Geometry: see drawing. Coordinates: mm, zero at the bounding-box minimum. A direction names the side the tool comes from. Give positions to 0.01 mm unless a question says otherwise; leave off trailing zeros. Order: outer loops, then holes, each group sorted by start corner. A loop starts at its lowest first (then second) coordinate and runs counter-clockwise, first axis right, second up. Notation, with made-up numbers: (-0.5, 15) -> (16.5, 15) arc R20 ccw to (16.5, 40) -> close; hole circle Ø2 at (22.5, -25.75). An arc over 180 degrees is marked (long way). Use one line per item in the form item = value. Start each with the question number.
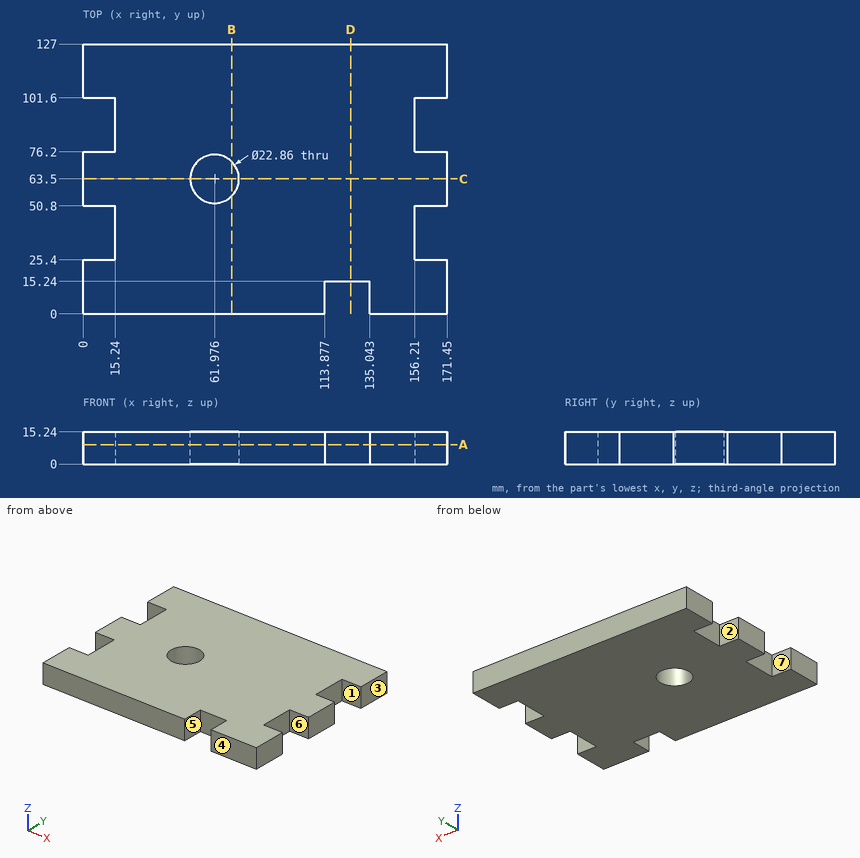
1) Cut plane A-A, the plane z = 9.25. Return the cut outline in (x, y).
2) Draft query along Y for the marked faces 1, 2, 3 and 4. Return one class per face: +Y half, -Y half, draft (parallel to the pull), parting line (faces both ways), or undercut.
3) Pin query (flat end, axial travel): pin 1 (1.5 mm diameter, centred on x = 37.5, z = 6.5, fed in from -Y); pin 2 (4.5 mm diameter, centred on y = 32.5, z = 4.5, fed in from -X); pin 3 (7.5 mm diameter, centred on y = 89, z = 11, fed in from +X). Return the tip coordinate at first contact, or that it passes through.
4) Cut plane D-D, the plane x = 126. Return the cut outline in (y, z).
5) Material intervals for probe 1 along Y at (x, z) = (8.5, 1.5); probe 2 along X at (y, z) = (81.5, 13.75); probe 3 along Y at (x, z) = (116, 7.25), sorted ascending.
6) Reachability of the marked faces 5, 6 and 7 from +Z, -Z, +X, -X, +Y, -Y: full face, straight path, thin tool, end or side. Return the list, or none.
7) Cut plane B-B, the plane x = 70. Return the cut outline in (y, z), plus the area to 3 significant figures.
8) Cut plane C-C, the plane y = 63.5. Return the cut outline in (x, z).
Output values:
q1.outline = (0, 0) -> (113.88, 0) -> (113.88, 15.24) -> (135.04, 15.24) -> (135.04, 0) -> (171.45, 0) -> (171.45, 25.4) -> (156.21, 25.4) -> (156.21, 50.8) -> (171.45, 50.8) -> (171.45, 76.2) -> (156.21, 76.2) -> (156.21, 101.6) -> (171.45, 101.6) -> (171.45, 127) -> (0, 127) -> (0, 101.6) -> (15.24, 101.6) -> (15.24, 76.2) -> (0, 76.2) -> (0, 50.8) -> (15.24, 50.8) -> (15.24, 25.4) -> (0, 25.4) -> close; hole circle Ø22.86 at (61.98, 63.5)
q2.face_1 = undercut
q2.face_2 = undercut
q2.face_3 = draft
q2.face_4 = -Y half
q3.pin_1 = 0
q3.pin_2 = 15.24
q3.pin_3 = 156.21
q4.outline = (15.24, 0) -> (127, 0) -> (127, 15.24) -> (15.24, 15.24) -> close
q5.probe_1 = 0 to 25.4, 50.8 to 76.2, 101.6 to 127
q5.probe_2 = 15.24 to 156.21
q5.probe_3 = 15.24 to 127
q6.face_5 = +Z, -Z, -Y
q6.face_6 = +Z, -Z, +X
q6.face_7 = +Z, -Z, -X
q7.outline = (0, 0) -> (55.36, 0) -> (55.36, 15.24) -> (0, 15.24) -> close; (71.64, 0) -> (127, 0) -> (127, 15.24) -> (71.64, 15.24) -> close
q7.area = 1,690 mm^2
q8.outline = (0, 0) -> (50.55, 0) -> (50.55, 15.24) -> (0, 15.24) -> close; (73.41, 0) -> (171.45, 0) -> (171.45, 15.24) -> (73.41, 15.24) -> close
